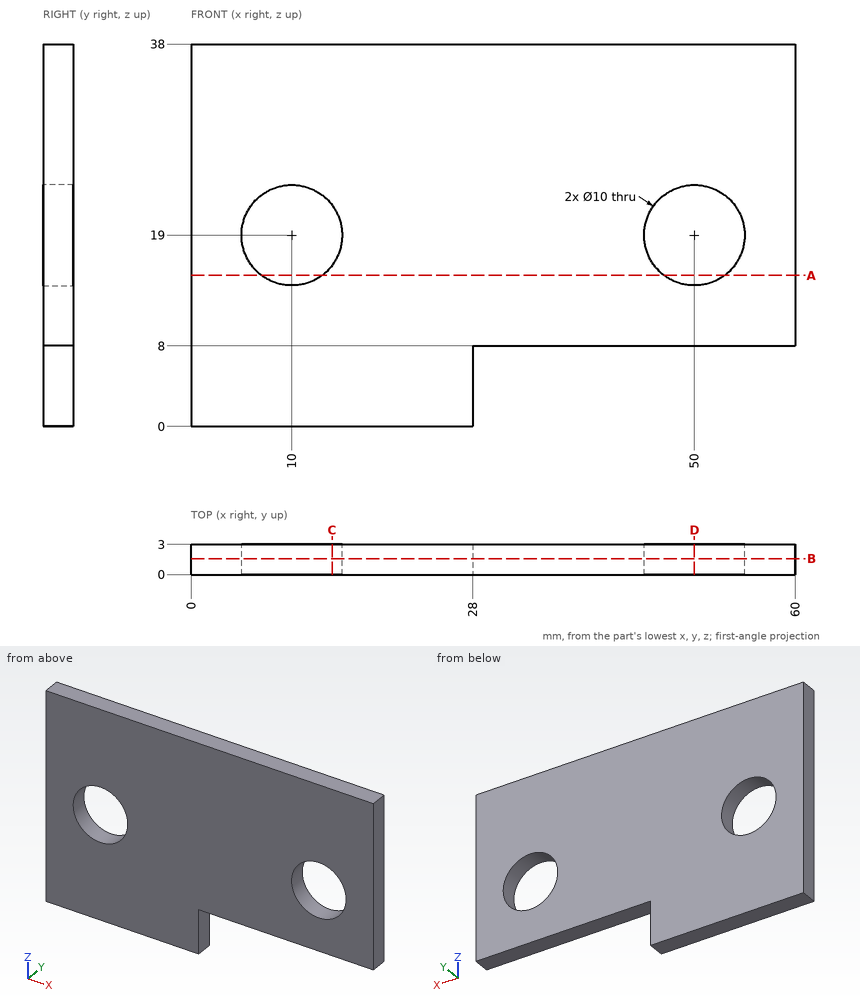
Geometry check sheet. Reference: drawing and pictorial views, mm from the part's lowest x, y, z. Round coordinates to 2 decimals unless told otherwise and drop trailing zeros. Loops run counter-clockwise (first coordinate to the right, second up) from the corner with the lowest first, then second, coordinate; pieces in that order, holes last.
1. Sectioned sample at C-C on x = 14. Record the boundary of the cut face in (y, z), and give its area (3 significant figures).
2. Scan lines: probe 1 along X at (y, z) = (1, 19); probe 2 along Z at (x, y) = (48.5, 1.7); probe 3 along X at (y, z) = (0.9, 23). Record each from-to range of solid material in increasing order.
3. Gauge pin test, flat ends, axial feed: pin 1 Ø9 at (x, z) = (50, 19) entering from -Y; pin 2 Ø0.9 at (x, y) = (51, 1) entering from -Z. Record the tip position at first contact, or that the pin passes through.
4. Sectioned sample at B-B on y = 1.6. Record the boundary of the cut face in (x, z).
5. Sectioned sample at A-A on z = 15. Record the boundary of the cut face in (x, y).
6. Sectioned sample at D-D on x = 50. Record the boundary of the cut face in (y, z).
Recorded:
1. outline: (0, 0) - (3, 0) - (3, 16) - (0, 16) - close; (0, 22) - (3, 22) - (3, 38) - (0, 38) - close
1. area: 96.0 mm2
2. probe 1: x = 0 to 5, 15 to 45, 55 to 60
2. probe 2: z = 8 to 14.23, 23.77 to 38
2. probe 3: x = 0 to 7, 13 to 47, 53 to 60
3. pin 1: passes through
3. pin 2: stops at z = 8
4. outline: (0, 0) - (28, 0) - (28, 8) - (60, 8) - (60, 38) - (0, 38) - close; hole circle Ø10 at (10, 19); hole circle Ø10 at (50, 19)
5. outline: (0, 0) - (7, 0) - (7, 3) - (0, 3) - close; (13, 0) - (47, 0) - (47, 3) - (13, 3) - close; (53, 0) - (60, 0) - (60, 3) - (53, 3) - close
6. outline: (0, 8) - (3, 8) - (3, 14) - (0, 14) - close; (0, 24) - (3, 24) - (3, 38) - (0, 38) - close
